Geometry check sheet. Reference: the model listing, model coordinates, mm. A direction names the side the tool comes from. Round coordinates to 2 decimals unless told otherwise and drop trailing zeros. Write each loop counter-clockwise with the first axis right and the second up, starting at its lowest first coordinate (ties: lowest second). Pieces come first, ordered by that corner, then holes. Notation, with made-up numbers: M 29,84.5 L 46,84.5 A8 cw 46,92.5 Z; hole C 69.25,-17.75 d11. An arc over 180 degrees is marked long. Answer as CSV lines item,"result". Start each with the question number.
```python
from build123d import *

# Parameters (mm, degrees)
SKETCH1_R           = 28.575
BOSS_EXTRUDE1_DEPTH = 6.35
SKETCH2_R           = 14.2875
BOSS_EXTRUDE2_DEPTH = 12.7
CUT_EXTRUDE1_DEPTH  = 20.05
SKETCH4_R           = 2
CUT_EXTRUDE2_DEPTH  = 7.35
FILLET1_R           = 1
SKETCH5_R           = 14.2875
CUT_EXTRUDE4_DEPTH  = 12.7
SKETCH7_R           = 0.25
CUT_EXTRUDE5_DEPTH  = 12.7


with BuildPart() as part:
    # Sketch1 → Boss-Extrude1 (new body)
    with BuildSketch(Plane.XY):
        Circle(SKETCH1_R)
    extrude(amount=BOSS_EXTRUDE1_DEPTH)

    # Sketch2 → Boss-Extrude2 (add)
    with BuildSketch(Plane.XY.offset(6.35)):
        Circle(SKETCH2_R)
    extrude(amount=BOSS_EXTRUDE2_DEPTH)

    # Sketch3 → Cut-Extrude1 (cut, through all)
    with BuildSketch(Plane.XY.offset(19.05)):
        Polygon((7.332348419, 0), (3.666174209, 6.35), (-3.666174209, 6.35), (-7.332348419, 0), (-3.666174209, -6.35), (3.666174209, -6.35), align=None)
    extrude(amount=-CUT_EXTRUDE1_DEPTH, mode=Mode.SUBTRACT)

    # Sketch4 → Cut-Extrude2 (cut, through all)
    with BuildSketch(Plane.XY.offset(6.35)):
        with Locations((25.4, 0)):
            Circle(SKETCH4_R)
        with Locations((12.7, -21.997045256)):
            Circle(SKETCH4_R)
        with Locations((-12.7, -21.997045256)):
            Circle(SKETCH4_R)
        with Locations((-25.4, 0)):
            Circle(SKETCH4_R)
        with Locations((-12.7, 21.997045256)):
            Circle(SKETCH4_R)
        with Locations((12.7, 21.997045256)):
            Circle(SKETCH4_R)
    extrude(amount=-CUT_EXTRUDE2_DEPTH, mode=Mode.SUBTRACT)

    # Fillet1
    fillet1_edges = [part.edges().sort_by_distance(p)[0] for p in [
        (5.499261314, -3.175, 19.05),
        (5.499261314, 3.175, 19.05),
        (0, 6.35, 19.05),
        (-5.499261314, 3.175, 19.05),
        (-5.499261314, -3.175, 19.05),
        (0, -6.35, 19.05),
    ]]
    fillet(fillet1_edges, radius=FILLET1_R)

    # Sketch5 → Cut-Extrude4 (cut)
    with BuildSketch(Plane.XY.offset(19.05)):
        Circle(SKETCH5_R)
    extrude(amount=-CUT_EXTRUDE4_DEPTH, mode=Mode.SUBTRACT)

    # Sketch7 → Cut-Extrude5 (cut)
    with BuildSketch(Plane.XY.offset(6.35)):
        with Locations((-3.666174209, 6.35)):
            Circle(SKETCH7_R)
        with Locations((3.666174209, 6.35)):
            Circle(SKETCH7_R)
        with Locations((7.332348419, 0)):
            Circle(SKETCH7_R)
        with Locations((3.666174209, -6.35)):
            Circle(SKETCH7_R)
        with Locations((-3.666174209, -6.35)):
            Circle(SKETCH7_R)
        with Locations((-7.332348419, 0)):
            Circle(SKETCH7_R)
    extrude(amount=-CUT_EXTRUDE5_DEPTH, mode=Mode.SUBTRACT)


solid = part.part
```
1) Section check A-A, the plane x = 0. Record the cut outline in (y, z) (3 decimals), plus the area to 3 significant figures.
2) Section check B-B, the plane x = -12.7. Record the cut outline in (y, z).
3) Section check D-D, the plane x = 25. Record the cut outline in (y, z).
4) Section check C-C, the plane z = 2.75. Give the number of separate pieces and of enclosed holes in the cut face, plus the area to 3 significant figures.
5) Access from +Z, -Z, +X, -X, +Y, -Y to the whole of each face (thin tool, end or side, straight path). Record for faces 1 (the flat face through (0, 7, 0)), 2 (the flat face through (0, -6.35, 3)).
6) Go/stop test with flat-tipped pins: pin 1 (6.5 mm diameter, centred on x = 12.7, y = 22, fed in from -Z); pin 2 (1.9 mm diameter, centred on x = 0.5, z = 4.5, fed in from +Y) (3 decimals); pin 3 (3 mm diameter, centred on y = 9, z = 4, fed in from -X); pin 4 (3 mm diameter, centred on x = -1, z = 2, fed in from -Y) (3 decimals). Record where each tip stops, or that it passes through.
7) Scan lines: line 1 (X direction, y = -21, z = 3); line 2 (Y direction, x = -6.5, z = 3); line 3 (Y direction, x = -3, z = 0.5). Record each from-to range of solid material in increasing order. Write a range as from..to.
8) Mould release check, pull along X, two halves, no side actions. Record for faces 3 (the flat face through (0, 7, 6.35)), 4 (the flat face through (5.475, -3.216, 3.219)), 5 (the cylindrical face through (-28.547, 1.256, 3.131)): released by +X, released by -X, zero draft, split by the parting line, or undercut.
Results:
1,outline,"M -28.575,0 L -6.35,0 L -6.35,6.35 L -28.575,6.35 Z; M 6.35,0 L 28.575,0 L 28.575,6.35 L 6.35,6.35 Z"
1,area,"282 mm^2"
2,outline,"M -25.6,0 L -24,0 L -24,6.35 L -25.6,6.35 Z; M -20,0 L 20,0 L 20,6.35 L -20,6.35 Z; M 24,0 L 25.6,0 L 25.6,6.35 L 24,6.35 Z"
3,outline,"M -13.84,0 L -1.96,0 L -1.96,6.35 L -13.84,6.35 Z; M 1.96,0 L 13.84,0 L 13.84,6.35 L 1.96,6.35 Z"
4,separate pieces,"1"
4,enclosed holes,"7"
4,area,"2,350 mm^2"
5,face 1,"-Z, +X, -X, +Y, -Y"
5,face 2,"+Z, -Z"
6,pin 1,"stops at z = 0"
6,pin 2,"stops at y = 28.575"
6,pin 3,"stops at x = -27.57"
6,pin 4,"stops at y = -28.575"
7,line 1,"x = -19.38..-14.43, -10.97..10.97, 14.43..19.38"
7,line 2,"y = -27.83..-1.44, 1.44..27.83"
7,line 3,"y = -28.42..-6.35, 6.35..28.42"
8,face 3,"zero draft"
8,face 4,"undercut"
8,face 5,"split by the parting line"
